Part print with two shaded views. Sizes in mm from the minimum x, y, z corner. Round coordinates to 2 decimals unless told otherwise and drop trailing zeros. Write each loop counter-clockwise with the first axis right and the second up, starting at its lowest first coordinate (ties: lowest second). Pieces come first, ordered by that corner, then holes.
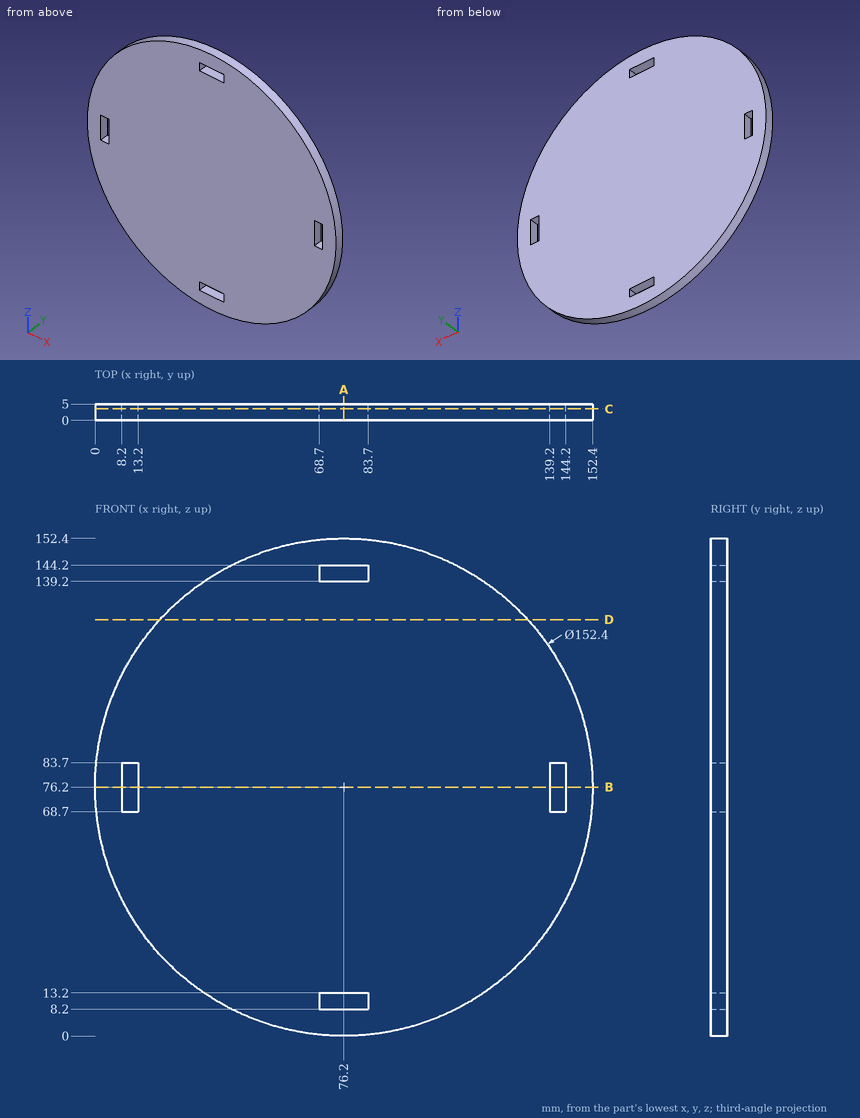
Q1. Drop flat-ended pins along their axis: pin 1 (1.5 mm diameter, centred on x = 141.5, y = 2.5, fed in from +Z); pin 2 (1 mm diameter, centred on x = 105.5, z = 85.5, fed in from -Y); pin 3 (1.5 mm diameter, centred on y = 3, z = 143, fed in from -X); pin 4 (1.5 mm diameter, centred on y = 3.5, z = 10, fed in from -X). Give the stop position or say it passes through.
Values follow:
pin 1: stops at z = 116.69
pin 2: stops at y = 0
pin 3: stops at x = 38.2
pin 4: stops at x = 37.18
Q2. Cut at C-C on y = 3.5. Write the cut outline in (x, z).
Values follow:
outline: circle Ø152.4 at (76.2, 76.2); hole (8.2, 68.7) - (13.2, 68.7) - (13.2, 83.7) - (8.2, 83.7) - close; hole (68.7, 8.2) - (83.7, 8.2) - (83.7, 13.2) - (68.7, 13.2) - close; hole (68.7, 139.2) - (83.7, 139.2) - (83.7, 144.2) - (68.7, 144.2) - close; hole (139.2, 68.7) - (144.2, 68.7) - (144.2, 83.7) - (139.2, 83.7) - close
Q3. Cut at B-B on z = 76.2. Write the cut outline in (x, y).
Values follow:
outline: (0, 0) - (8.2, 0) - (8.2, 5) - (0, 5) - close; (13.2, 0) - (139.2, 0) - (139.2, 5) - (13.2, 5) - close; (144.2, 0) - (152.4, 0) - (152.4, 5) - (144.2, 5) - close
Q4. Cut at A-A on x = 76.2. Write the cut outline in (y, z).
Values follow:
outline: (0, 0) - (5, 0) - (5, 8.2) - (0, 8.2) - close; (0, 13.2) - (5, 13.2) - (5, 139.2) - (0, 139.2) - close; (0, 144.2) - (5, 144.2) - (5, 152.4) - (0, 152.4) - close
Q5. Cut at D-D on z = 127.5. Write the cut outline in (x, y).
Values follow:
outline: (19.86, 0) - (132.54, 0) - (132.54, 5) - (19.86, 5) - close
Q6. Wall check: L1, parallel to Z at x = 76.5, y = 4.3; L2, parallel to X at y = 4.7, z = 142.5; L3, parallel to X at y = 3.4, z = 13. Give the ranges that are in metal, low to high.
Values follow:
L1: z = 0 to 8.2, 13.2 to 139.2, 144.2 to 152.4
L2: x = 38.64 to 68.7, 83.7 to 113.76
L3: x = 33.63 to 68.7, 83.7 to 118.77
